Geometry: final body of the model. Coordinates: model frame, mm. Face numbers are marked on the shaded views. A direction names the side the tool comes from. Round coordinates to 2 decimals unless told otherwise and drop trailing zeros. Loops run counter-clockwise (first coordinate to the right, second up) from the corner with the lowest first, then second, coordinate; pieces in that order, holes last. Notation, with made-up numbers: (4.5, 60.5) - (33.5, 60.5) arc R17 cw to (33.5, 73.5) - close; hole circle Ø5 at (73.25, 87). An arc over 180 degrees is marked (long way). Write item = value, one per line. Start each with the question number.
Item 1: Line query: line 1 (X direction, y = -1, z = 8); line 2 (X direction, y = 11.5, z = 35); line 3 (Z direction, x = -22, y = 3.5). Output: solid intervals per line, ascending. Write a range as from..to.
Item 2: Access query for the marked faces 1, 2, 3 and 4. Directions: +Z, -Z, +X, -X, +Y, -Y. A direction counts if a zero-diameter tool reaches every point of the face in a straight line with its end or side. Return the directions, or none.
Item 3: Section A-A (z = 49.5). Return loops of the section in (x, y).
Item 4: Section C-C (y = -10.75). Return loops of the section in (x, z), plus the area to 3 significant figures.
Item 5: Section D-D (z = 23). Return loops of the section in (x, y).
Item 6: Section B-B (x = 17). Return loops of the section in (y, z).
Item 7: First-contact query: pin 1 (13 mm diameter, centred on y = 4.5, z = 54.5, fed in from -X); pin 2 (7.5 mm diameter, centred on y = 3.5, z = 19.5, fed in from -X); pin 3 (0.5 mm diameter, centred on x = 1.5, y = 4.5, fed in from +Z); pin 4 (5 mm diameter, centred on x = 9, z = 5.5, fed in from -Y). Flat tips, straight axial feed; report the tip coordinate or a pass-through.
Item 8: Draft query along X for the marked faces 5, 6 and 7. Return one class per face: pulls with the +X half, pulls with the -X half, needs draft (parallel to the pull), parting line crosses it, or undercut.
from build123d import *

# Parameters (mm, degrees)
F1_DEPTH = 12.5
F2_R     = 5
F3_R     = 2.5
F4_R     = 1


with BuildPart() as f1:
    # F0 (on Front) → F1 (new body, symmetric)
    with BuildSketch(Plane.XZ):
        Polygon((0, 0), (-44.5, 0), (-44.5, 15), (-49.5, 15), (-49.5, -5), (-44.5, -5), (0, -5), (5, -5), (5, 39), (34, 39), (34, 47.355823), (8, 58), (3, 58), (3, 45), (0, 45), align=None)
        Polygon((29, 44), (8, 44), (8, 52.59722), align=None, mode=Mode.SUBTRACT)
    extrude(amount=F1_DEPTH, both=True)

    # F2
    f2_edges = [f1.edges().sort_by_distance(p)[0] for p in [
        (34, 0, 39),
    ]]
    fillet(f2_edges, radius=F2_R)

    # F3
    f3_edges = [f1.edges().sort_by_distance(p)[0] for p in [
        (5, 0, -5),
        (-49.5, 0, -5),
        (-49.5, 0, 15),
        (34, 0, 47.355823),
        (5, 0, 39),
    ]]
    fillet(f3_edges, radius=F3_R)

    # F4
    f4_edges = [f1.edges().sort_by_distance(p)[0] for p in [
        (3, 0, 45),
        (0, 0, 45),
        (0, 0, 0),
        (-44.5, 0, 0),
    ]]
    fillet(f4_edges, radius=F4_R)


solid = f1.part
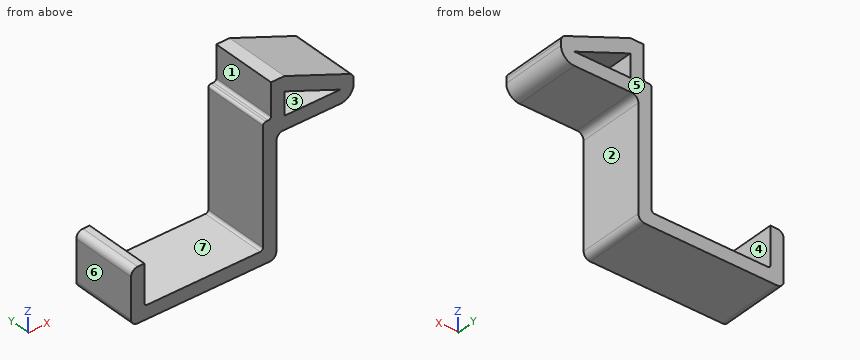
Taken from the geometry:
q1.line_1 = -49.5..-44.5, 0..5
q1.line_2 = 0..5
q1.line_3 = -5..0
q2.face_1 = +Z, -X, +Y, -Y
q2.face_2 = -Z, +X, +Y, -Y
q2.face_3 = +Y, -Y
q2.face_4 = +Z, +Y, -Y
q3.outline = (3, -12.5) - (8, -12.5) - (8, 12.5) - (3, 12.5) - close; (15.57, -12.5) - (28.76, -12.5) - (28.76, 12.5) - (15.57, 12.5) - close
q4.outline = (-49.5, -2.5) arc R2.5 ccw to (-47, -5) - (2.5, -5) arc R2.5 ccw to (5, -2.5) - (5, 36.5) arc R2.5 cw to (7.5, 39) - (29, 39) arc R5 ccw to (34, 44) - (34, 45.68) arc R2.5 ccw to (32.45, 47.99) - (8, 58) - (3, 58) - (3, 46) arc R1 cw to (2, 45) - (1, 45) arc R1 ccw to (0, 44) - (0, 1) arc R1 cw to (-1, 0) - (-43.5, 0) arc R1 cw to (-44.5, 1) - (-44.5, 15) - (-47, 15) arc R2.5 ccw to (-49.5, 12.5) - close; hole (8, 44) - (29, 44) - (8, 52.6) - close
q4.area = 913 mm^2
q5.outline = (0, -12.5) - (5, -12.5) - (5, 12.5) - (0, 12.5) - close
q6.outline = (-12.5, 39) - (12.5, 39) - (12.5, 44) - (-12.5, 44) - close; (-12.5, 48.91) - (12.5, 48.91) - (12.5, 54.32) - (-12.5, 54.32) - close
q7.pin_1 = 3
q7.pin_2 = 0
q7.pin_3 = 45
q7.pin_4 = through
q8.face_5 = needs draft
q8.face_6 = pulls with the -X half
q8.face_7 = undercut
